```python
from build123d import *

# Parameters (mm, degrees)
SKETCH1_W               = 18.9
SKETCH1_H               = 18.9
SKETCH1_R               = 1.255147878
BOSS_EXTRUDE1_DEPTH     = 4
FILLET1_R               = 3.5
BOSS_EXTRUDE2_DEPTH     = 7.2
SKETCH3_R               = 1.5
CUT_EXTRUDE1_DEPTH      = 7.2
CUT_EXTRUDE2_DEPTH      = 1
CUT_EXTRUDE2_DEPTH_BACK = 1
CUT_EXTRUDE3_START      = -4
CUT_EXTRUDE3_DEPTH      = 4
SKETCH6_W               = 8.351743046
SKETCH6_H               = 2
CUT_EXTRUDE4_DEPTH      = 7.2
SKETCH7_W               = 6.001336377
SKETCH7_H               = 3.250686631
CUT_EXTRUDE5_DEPTH      = 4


with BuildPart() as part:
    # Sketch1 → Boss-Extrude1 (new body)
    with BuildSketch(Plane(origin=(0, 0, 0), x_dir=(1, 0, 0), z_dir=(0, 1, 0))):
        Rectangle(SKETCH1_W, SKETCH1_H)
        with Locations(Location((-6.75, 6.75, 0), (0, 0, 270))):
            Circle(SKETCH1_R, mode=Mode.SUBTRACT)
        with Locations(Location((6.75, 6.75, 0), (0, 0, 270))):
            Circle(SKETCH1_R, mode=Mode.SUBTRACT)
        with Locations(Location((6.75, -6.75, 0), (0, 0, 270))):
            Circle(SKETCH1_R, mode=Mode.SUBTRACT)
        with Locations(Location((-6.75, -6.75, 0), (0, 0, 270))):
            Circle(SKETCH1_R, mode=Mode.SUBTRACT)
    extrude(amount=BOSS_EXTRUDE1_DEPTH)

    # Fillet1
    fillet1_edges = [part.edges().sort_by_distance(p)[0] for p in [
        (-9.45, 2, 9.45),
        (-9.45, 2, -9.45),
        (9.45, 2, -9.45),
        (9.45, 2, 9.45),
    ]]
    fillet(fillet1_edges, radius=FILLET1_R)

    # Sketch2 → Boss-Extrude2 (add)
    with BuildSketch(Plane(origin=(0, 4, 0), x_dir=(1, 0, 0), z_dir=(0, 1, 0))):
        with BuildLine():
            Line((1.89565101, -6.265449543), (-1.89565101, -6.265449543))
            ThreePointArc((-1.89565101, -6.265449543), (0, 6.545941546), (1.89565101, -6.265449543))
        make_face()
        with BuildLine():
            Line((1.42, -2.901120473), (-1.42, -2.901120473))
            ThreePointArc((-1.42, -2.901120473), (0, 3.23), (1.42, -2.901120473))
        make_face(mode=Mode.SUBTRACT)
    extrude(amount=BOSS_EXTRUDE2_DEPTH)

    # Sketch3 → Cut-Extrude1 (cut)
    with BuildSketch(Plane.XY.offset(6.265449543)):
        with Locations((0, 7.6)):
            Circle(SKETCH3_R)
    extrude(amount=-CUT_EXTRUDE1_DEPTH, mode=Mode.SUBTRACT)

    # Sketch4 → Cut-Extrude2 (cut, two sides: drawn at the far end of the back side and taken through both)
    with BuildSketch(Plane(origin=(0, 0, 4.583285008), x_dir=(-1, 0, 0), z_dir=(0, 0, -1)).offset(-CUT_EXTRUDE2_DEPTH_BACK)):
        Polygon((-2.765, 9.196373494), (-2.765, 6.003626506), (0, 4.407253011), (2.765, 6.003626506), (2.765, 9.196373494), (0, 10.792746989), align=None)
        Polygon((2.765, 11.723212655), (-2.765, 11.723212655), (-2.765, 9.196373494), (0, 10.792746989), (2.765, 9.196373494), align=None)
    extrude(amount=CUT_EXTRUDE2_DEPTH + CUT_EXTRUDE2_DEPTH_BACK, mode=Mode.SUBTRACT)

    # Sketch5 → Cut-Extrude3 (cut)
    with BuildSketch(Plane(origin=(0, 4, 0), x_dir=(1, 0, 0), z_dir=(0, 1, 0)).offset(CUT_EXTRUDE3_START)):
        with BuildLine():
            Line((-1.42, -2.901120473), (1.42, -2.901120473))
            ThreePointArc((1.42, -2.901120473), (0, 3.23), (-1.42, -2.901120473))
        make_face()
    extrude(amount=CUT_EXTRUDE3_DEPTH, mode=Mode.SUBTRACT)

    # Sketch6 → Cut-Extrude4 (cut)
    with BuildSketch(Plane(origin=(0, 11.2, 0), x_dir=(1, 0, 0), z_dir=(0, 1, 0))):
        with Locations((0, 6.040976864)):
            Rectangle(SKETCH6_W, SKETCH6_H)
    extrude(amount=-CUT_EXTRUDE4_DEPTH, mode=Mode.SUBTRACT)

    # Sketch7 → Cut-Extrude5 (cut)
    with BuildSketch(Plane(origin=(0, 4, 0), x_dir=(1, 0, 0), z_dir=(0, 1, 0))):
        with Locations((0.224673796, 6.666320179)):
            Rectangle(SKETCH7_W, SKETCH7_H)
    extrude(amount=-CUT_EXTRUDE5_DEPTH, mode=Mode.SUBTRACT)


solid = part.part
```
Here's how the part is built. I have some questions about the finished solid (model axes, mm). A direction names the side the tool comes from. Round coordinates to 2 decimals unless told otherwise and drop trailing zeros. Order: outer loops, then holes, each group sorted by start corner. A loop starts at its lowest first (then second) coordinate and runs counter-clockwise, first axis right, second up. Notation, with made-up numbers: M 79.25,-7.5 L 104.25,-7.5 A22 ccw 104.25,20.5 Z; hole C 66,-7 d11. An arc over 180 degrees is marked long. Use CSV: the item, a comma, the result in double quotes.
1) I want a section at A-A (z = 0). List the corners of the cut face in (x, y) for me, then the cut area to 3 significant figures.
Taken from the geometry:
outline,"M -9.45,0 L -3.23,0 L -3.23,11.2 L -6.55,11.2 L -6.55,4 L -9.45,4 Z; M 3.23,0 L 9.45,0 L 9.45,4 L 6.55,4 L 6.55,11.2 L 3.23,11.2 Z"
area,"97.5 mm^2"
2) I'm going to push flat-ended pins straight in: P1, Ø2, axis at y = 9, z = 4.5, coming from the -X side; P2, Ø2, axis at x = -6.75, z = 6.75, coming from the +Y side; P3, Ø1.5, axis at x = 5, y = 7.5, coming from the +Z side; P4, Ø1.7, axis at x = -1, y = 9.5, coming from the +Z side. Where does each tip first touch, or does it pass through?
Taken from the geometry:
P1,"x = -5.53"
P2,"through"
P3,"z = 4.98"
P4,"z = 6.27"
3) I need wall thicknesses on line 1 along Z through (x, y) = (0, 3); line 2 along X through (y, z) = (2.25, 6.5); line 3 along Y through (x, z) = (0, 3.2). Which ranges of each line are inside material? Lowest first, please. Write a range as [from, to].
Taken from the geometry:
line 1,"[-9.45, -8.29], [-5.04, -3.23], [2.9, 9.45]"
line 2,"[-9.41, -7.98], [-5.52, 5.52], [7.98, 9.41]"
line 3,"[0, 6.1], [9.1, 11.2]"
4) I want a section at D-D (y = 7.6). List the corners of the cut face in (x, z) for me (3 decimals), then the cut area to 3 significant figures.
Taken from the geometry:
outline,"M -4.176,-5.041 L 4.176,-5.041 A6.546 ccw 1.896,6.265 L 1.5,6.265 L 1.5,5.583 L 2.765,5.583 L 2.765,3.583 L 1.5,3.583 L 1.5,2.861 A3.23 cw long -1.5,2.861 L -1.5,3.583 L -2.765,3.583 L -2.765,5.583 L -1.5,5.583 L -1.5,6.265 L -1.896,6.265 A6.546 ccw Z"
area,"78.0 mm^2"
5) On a 3-axis mill with a long thin cutter (end or side, diameter ignored), from which of +Z, -Z, +X, -X, +Y, -Y can I reach the whole of each face in a straight line? I mean faces 4 (the flat face through (-1.363, 5.194, 4.597)), 5 (the flat face through (-3, 11.2, 2)), 6 (the cylindrical face through (6.436, 7.55, 1.197)), 7 (the flat face through (0, 10, 2.901)), 8 (the flat face through (9.45, 2, 0)). Say none if no direction works.
Taken from the geometry:
face 4,"+Y"
face 5,"+Z, -Z, +X, -X, +Y"
face 6,"+X, +Y"
face 7,"+Y, -Y"
face 8,"+Z, -Z, +X, +Y, -Y"
6) If we mould it in two halves opening along X, with no side actions, what happens to faces 1 (the cylindrical face through (-6.396, 7.55, 1.391)), 2 (the flat face through (0, 2, 9.45)), 3 (the flat face through (1.402, 5.217, 4.597))? For each: pulls with the +X half, pulls with the -X half, needs draft (parallel to the pull), parting line crosses it, or undercut.
Taken from the geometry:
face 1,"pulls with the -X half"
face 2,"needs draft"
face 3,"undercut"
7) I want a section at B-B (y = 2.5). List the corners of the cut face in (x, z) for me, then the cut area to 3 significant figures.
Taken from the geometry:
outline,"M -9.45,-5.95 A3.5 ccw -5.95,-9.45 L 5.95,-9.45 A3.5 ccw 9.45,-5.95 L 9.45,5.95 A3.5 ccw 5.95,9.45 L -5.95,9.45 A3.5 ccw -9.45,5.95 Z; hole C -6.75,-6.75 d2.51; hole C -6.75,6.75 d2.51; hole M -2.78,-8.29 L 3.23,-8.29 L 3.23,-5.04 L -2.78,-5.04 Z; hole M -1.42,2.9 A3.23 ccw long 1.42,2.9 Z; hole C 6.75,-6.75 d2.51; hole C 6.75,6.75 d2.51"
area,"275 mm^2"
8) I want a section at C-C (z = 3.25). List the corners of the cut face in (x, y) for me, then the cut area to 3 significant figures.
Taken from the geometry:
outline,"M -9.45,0 L 9.45,0 L 9.45,4 L 5.68,4 L 5.68,11.2 L -5.68,11.2 L -5.68,4 L -9.45,4 Z; hole C 0,7.6 d3"
area,"150 mm^2"
